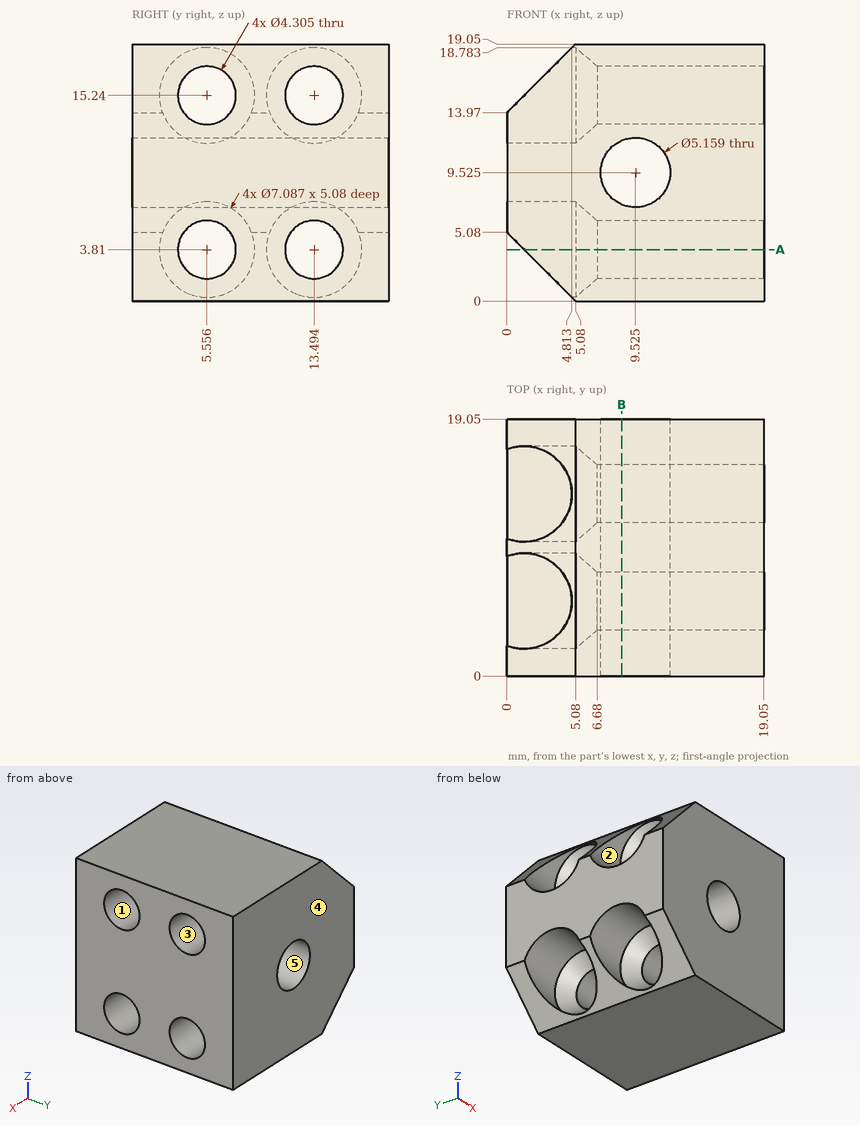
Here's the drawing with two shaded views (mm, measured from the low corner). I have some questions. A direction names the side the tool comes from. Coordinates: 2 decimals unless noted, no trailing zeros. Write each loop counter-clockwise with the first axis right and the second up, starting at its lowest first coordinate (ties: lowest second). Pieces come first, ordered by that corner, then holes. Notation, with made-up numbers: (44, -8) -> (80, -8) arc R25 ccw to (80, 14) -> close; hole circle Ø7 at (35, -2.75). An arc over 180 degrees is marked (long way). Use a Markdown table: item, result. Add a question column.
(1) If we section it at A-A, the plane z = 3.81: Write out the boundary of the cut face in (x, y).
(2) Please list where these lines run through material, in increasing order: line 1 (Y direction, x = 3, z = 15.24); line 2 (Y direction, x = 14.5, z = 15.24); line 3 (Z direction, x = 14.25, y = 6).
(3) We'd pull the mould along Y, two halves only. Please class the marked faces 3, 4 and 5: +Y half, -Y half, draft (parallel to the pull), parting line (faces both ways), or undercut.
(4) If we section it at B-B, the plane x = 8.5: State how many separate pieces and enclosed holes the cut face has.
(5) I'm going to push flat-ended pins straight in: P1, Ø7, axis at y = 13.49, z = 3.81, coming from the +X side; P2, Ø3.5, axis at y = 13.49, z = 15.24, coming from the -X side; P3, Ø6.5, axis at y = 13.49, z = 3.81, coming from the -X side. Where does each tip first touch, or does it pass through?
(6) For the marked faces 1 and 2, which set-ups out of +Z, -Z, +X, -X, +Y, -Y let a thin tool reach every point of the face, with its end or its side?
Outcome:
| question | item | result |
|---|---|---|
| 1 | outline | (1.27, 0) -> (19.05, 0) -> (19.05, 3.4) -> (6.68, 3.4) -> (5.08, 2.01) -> (1.27, 2.01) -> close; (1.27, 9.1) -> (5.08, 9.1) -> (6.68, 7.71) -> (19.05, 7.71) -> (19.05, 11.34) -> (6.68, 11.34) -> (5.08, 9.95) -> (1.27, 9.95) -> close; (1.27, 17.04) -> (5.08, 17.04) -> (6.68, 15.65) -> (19.05, 15.65) -> (19.05, 19.05) -> (1.27, 19.05) -> close |
| 2 | line 1 | y = 0 to 2.01, 9.1 to 9.95, 17.04 to 19.05 |
| 2 | line 2 | y = 0 to 3.4, 7.71 to 11.34, 15.65 to 19.05 |
| 2 | line 3 | z = 0 to 1.7, 5.92 to 13.13, 17.35 to 19.05 |
| 3 | face 3 | undercut |
| 3 | face 4 | +Y half |
| 3 | face 5 | draft |
| 4 | separate pieces | 2 |
| 4 | enclosed holes | 4 |
| 5 | P1 | stops at x = 19.05 |
| 5 | P2 | passes through |
| 5 | P3 | stops at x = 5.41 |
| 6 | face 1 | +X, -X |
| 6 | face 2 | -X |
